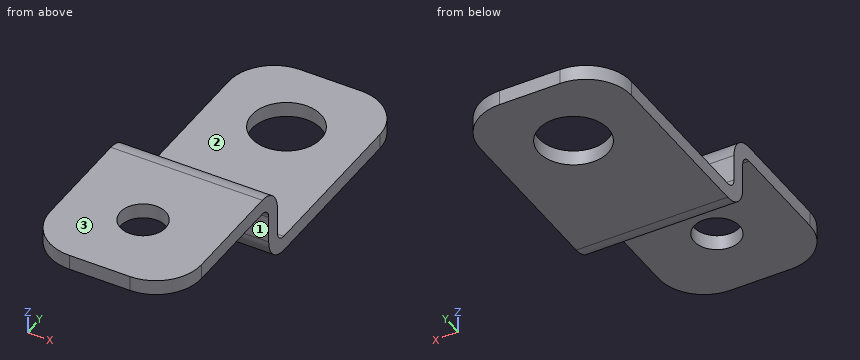
from build123d import *

# Parameters (mm, degrees)
SKETCH1_W          = 10
SKETCH1_H          = 14.057527786
SKETCH1_R          = 2.287307526
BASE_FLANGE1_DEPTH = 1
EDGE_FLANGE1_DEPTH = 10
EDGE_FLANGE2_DEPTH = 10
SKETCH12_R         = 1.5
CUT_EXTRUDE1_DEPTH = 2
FILLET1_R          = 3


# Sheet-metal steps are written as plain solids
with BuildPart() as part:
    # Sketch1 → Base-Flange1 (new body)
    with BuildSketch(Plane.XY):
        with Locations((-509.974194853, -21.379047402)):
            Rectangle(SKETCH1_W, SKETCH1_H)
        with Locations((-509.974194853, -19.4)):
            Circle(SKETCH1_R, mode=Mode.SUBTRACT)
    extrude(amount=BASE_FLANGE1_DEPTH)

    # Edge-Flange1 section (across the edge) → Edge-Flange1 (add)
    with BuildSketch(Plane(origin=(-514.974194853, -29.144411295, 1), x_dir=(0, 1, 0), z_dir=(1, 0, 0))):
        with BuildLine():
            Line((-1, 0.7366), (-1, 2.5))
            Line((-1, 2.5), (0, 2.5))
            Line((0, 2.5), (0, 0.7366))
            ThreePointArc((0, 0.7366), (0.215745145, 0.215745145), (0.7366, 0))
            Line((0.7366, 0), (0.7366, -1))
            ThreePointArc((0.7366, -1), (-0.491361636, -0.491361636), (-1, 0.7366))
        make_face()
    extrude(amount=EDGE_FLANGE1_DEPTH)

    # Edge-Flange2 section (across the edge) → Edge-Flange2 (add)
    with BuildSketch(Plane(origin=(-504.974194853, -30.144411295, 4.2366), x_dir=(0, 0, -1), z_dir=(-1, 0, 0))):
        with BuildLine():
            Line((-1, 0.7366), (-1, 10.7366))
            Line((-1, 10.7366), (0, 10.7366))
            Line((0, 10.7366), (0, 0.7366))
            ThreePointArc((0, 0.7366), (0.215745145, 0.215745145), (0.7366, 0))
            Line((0.7366, 0), (0.7366, -1))
            ThreePointArc((0.7366, -1), (-0.491361636, -0.491361636), (-1, 0.7366))
        make_face()
    extrude(amount=EDGE_FLANGE2_DEPTH)

    # Sketch12 → Cut-Extrude1 (cut)
    with BuildSketch(Plane(origin=(0, 0, 4.2366), x_dir=(-1, 0, 0), z_dir=(0, 0, -1))):
        with Locations((509.974194853, -35.881011295)):
            Circle(SKETCH12_R)
    extrude(amount=-CUT_EXTRUDE1_DEPTH, mode=Mode.SUBTRACT)

    # Fillet1
    fillet1_edges = [part.edges().sort_by_distance(p)[0] for p in [
        (-504.974194853, -40.881011295, 4.7366),
        (-514.974194853, -40.881011295, 4.7366),
        (-514.974194853, -14.350283509, 0.5),
        (-504.974194853, -14.350283509, 0.5),
    ]]
    fillet(fillet1_edges, radius=FILLET1_R)


solid = part.part
Geometry check sheet. Reference: the model listing, model coordinates, mm. Face numbers are marked on the shaded views. A direction names the side the tool comes from. Round coordinates to 2 decimals unless told otherwise and drop trailing zeros. Order: outer loops, then holes, each group sorted by start corner. A loop starts at its lowest first (then second) coordinate and runs counter-clockwise, first axis right, second up. Notation, with made-up numbers: (33, 45.5) - (66, 45.5) arc R10 cw to (66, 62.5) - close; hole circle Ø4 at (39, 19.25). An arc over 180 degrees is marked (long way). One line per question, with ' | ' between items. Start each with the question number.
(1) Sectioned sample at B-B on x = -506. Record the cut outline in (y, z).
(2) Thickness scan on L1, parallel to Z at x = -506, y = -20.75; L2, parallel to Z at x = -508, y = -33.25; L3, parallel to X at y = -21.5, z = 0.95. Record the ranges inside material, lowest first. Write a range as [from, to].
(3) Sectioned sample at A-A on y = -19.4. Record the cut outline in (x, z), and give its area (3 significant figures).
(4) Sectioned sample at C-C on x = -509.5. Record the cut outline in (y, z).
(5) Sectioned sample at D-D on y = -26. Record the cut outline in (x, z).
(6) Depth check by flat-ended pin: pin 1 Ø3 at (x, y) = (-511.5, -35.5) entering from -Z; pin 2 Ø1.4 at (x, z) = (-508, 3) entering from +Y; pin 3 Ø0.5 at (x, z) = (-508, 2.5) entering from -Y. Enter the tip coordinate at first touch or a pass-through.
(7) Access from +Z, -Z, +X, -X, +Y, -Y to the whole of each face (thin tool, end or side, straight path). Record for the marked faces 1, 2 and 3.
Conclusion:
1) outline: (-40.14, 4.24) - (-30.88, 4.24) arc R0.74 cw to (-30.14, 3.5) - (-30.14, 1.74) arc R1.74 ccw to (-28.41, 0) - (-15.09, 0) - (-15.09, 1) - (-28.41, 1) arc R0.74 cw to (-29.14, 1.74) - (-29.14, 3.5) arc R1.74 ccw to (-30.88, 5.24) - (-40.14, 5.24) - close
2) L1: z = [0, 1] | L2: z = [4.24, 5.24] | L3: x = [-514.97, -510.88], [-509.07, -504.97]
3) outline: (-514.97, 0) - (-512.26, 0) - (-512.26, 1) - (-514.97, 1) - close; (-507.69, 0) - (-504.97, 0) - (-504.97, 1) - (-507.69, 1) - close | area: 5.43 mm2
4) outline: (-40.88, 4.24) - (-37.3, 4.24) - (-37.3, 5.24) - (-40.88, 5.24) - close; (-34.46, 4.24) - (-30.88, 4.24) arc R0.74 cw to (-30.14, 3.5) - (-30.14, 1.74) arc R1.74 ccw to (-28.41, 0) - (-21.64, 0) - (-21.64, 1) - (-28.41, 1) arc R0.74 cw to (-29.14, 1.74) - (-29.14, 3.5) arc R1.74 ccw to (-30.88, 5.24) - (-34.46, 5.24) - close; (-17.16, 0) - (-14.35, 0) - (-14.35, 1) - (-17.16, 1) - close
5) outline: (-514.97, 0) - (-504.97, 0) - (-504.97, 1) - (-514.97, 1) - close
6) pin 1: stops at z = 4.24 | pin 2: stops at y = -29.14 | pin 3: stops at y = -30.14
7) face 1: -Z, +X, -X, -Y | face 2: +Z, +X, -X, +Y | face 3: +Z, +X, -X, +Y, -Y
